Part model, mm, in its own coordinate system. Give positions to 0.01 mm unless a question says otherwise; leave off trailing zeros. Order: outer loops, then holes, each group sorted by start corner. A loop starts at its lowest first (then second) coordinate and runs counter-clockwise, first axis right, second up.
1. Mould opens along X. For faces 1 (the flat face through (0, 35, 40)), 2 (the flat face through (0, 65, 0)), 3 (the cylindrical face through (-37.15, 34.51, 36.99)), 4 (the cylindrical face through (-4.88, 67.54, -1.08)) say: +X half, -X half, draft (parallel to the pull), parting line (faces both ways), or undercut.
2. Slice it at A-A on x = 35. List the corners of the cut face in (y, z).
3. Drop a flat-ended pin along its axis: pin 1 Ø6 at (x, z) = (-2, -26) entering from -Y. Give the stop position or say it passes through.
4. Probe line 1 (X direction, y = 67.45, z = 0); line 2 (Z direction, x = 30.5, y = 43.5); line 3 (X direction, y = 13.5, z = 32). List the from-to ranges inside material, lowest first.
from build123d import *

# Parameters (mm, degrees)
BOSS_EXTRUDE1_DEPTH = 70
SKETCH2_R           = 5
CUT_EXTRUDE1_DEPTH  = 5


with BuildPart() as part:
    # Sketch1 → Boss-Extrude1 (new body)
    with BuildSketch(Plane(origin=(0, 0, 0), x_dir=(1, 0, 0), z_dir=(0, 1, 0))):
        with BuildLine():
            Line((-30, -40), (30, -40))
            ThreePointArc((30, -40), (37.071067812, -37.071067812), (40, -30))
            Line((40, -30), (40, 30))
            ThreePointArc((40, 30), (37.071067812, 37.071067812), (30, 40))
            Line((30, 40), (-30, 40))
            ThreePointArc((-30, 40), (-37.071067812, 37.071067812), (-40, 30))
            Line((-40, 30), (-40, -30))
            ThreePointArc((-40, -30), (-37.071067812, -37.071067812), (-30, -40))
        make_face()
    extrude(amount=BOSS_EXTRUDE1_DEPTH)

    # Sketch2 → Cut-Extrude1 (cut)
    with BuildSketch(Plane(origin=(0, 70, 0), x_dir=(1, 0, 0), z_dir=(0, 1, 0))):
        with Locations(Location((0, 0, 0), (0, 0, 270))):
            Circle(SKETCH2_R)
    extrude(amount=-CUT_EXTRUDE1_DEPTH, mode=Mode.SUBTRACT)


solid = part.part
Data:
1. face 1: draft
1. face 2: undercut
1. face 3: -X half
1. face 4: undercut
2. outline: (0, -38.66) - (70, -38.66) - (70, 38.66) - (0, 38.66) - close
3. pin 1: stops at y = 0
4. line 1: x = -40 to -5, 5 to 40
4. line 2: z = -39.99 to 39.99
4. line 3: x = -39.8 to 39.8
